Verification items for this drawing (mm, ordinates from the low corner). Coordinates: 2 decimals unless noted, no trailing zeros. One line per item, written item: value. Start each with the question number.
1) Scan lines: line 1 along Z through (x, y) = (170, 0.65); line 2 along X through (y, z) = (0.6, 115); line 3 along X through (y, z) = (1.5, 5). Record each from-to range of solid material in increasing order. Write a range as [from, to].
2) Gauge pin test, flat ends, axial feed: P1, Ø5, axis at x = 100.5, z = 70.5, coming from the -Y side; P2, Ø2.5, axis at x = 170, z = 115, coming from the +Y side. Record the tip position at first contact, or that the pin passes through.
3) Draft check along Y on the marked faces 1 and 2. Enter one of: +Y half, -Y half, draft (parallel to the pull), parting line (faces both ways), or undercut.
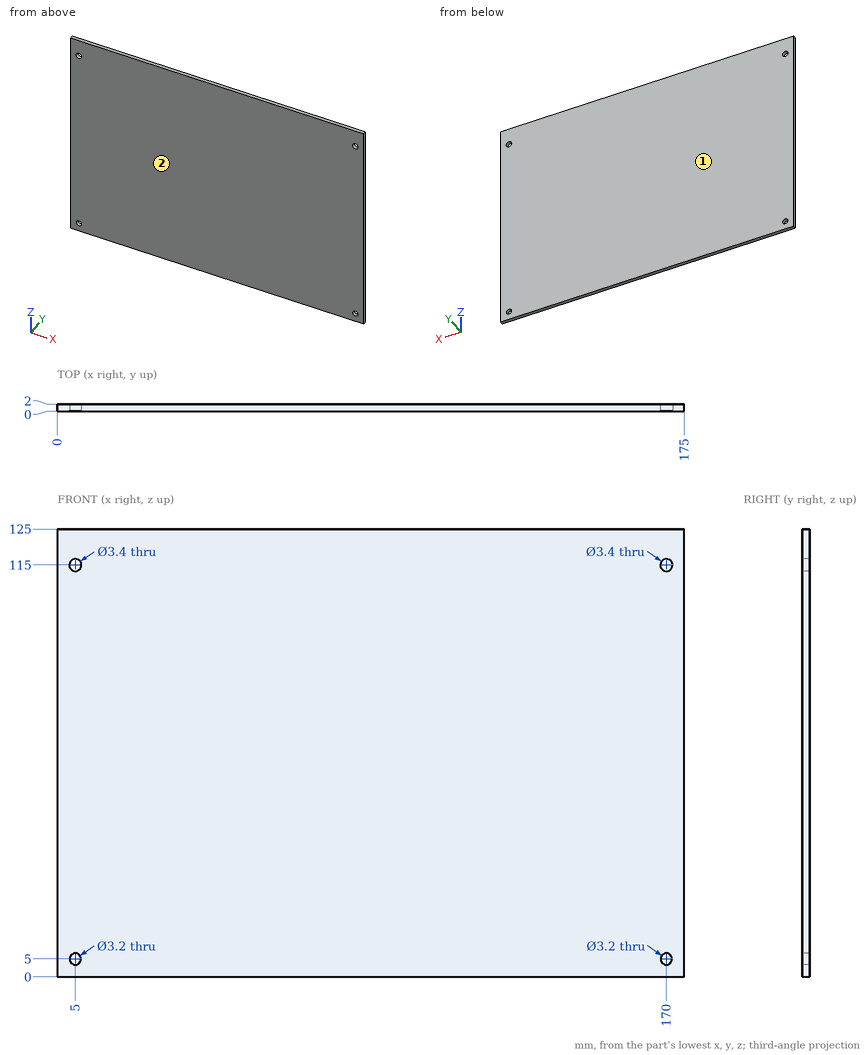
Answers:
1. line 1: z = [0, 3.4], [6.6, 113.3], [116.7, 125]
1. line 2: x = [0, 3.3], [6.7, 168.3], [171.7, 175]
1. line 3: x = [0, 3.4], [6.6, 168.4], [171.6, 175]
2. P1: stops at y = 0
2. P2: passes through
3. face 1: +Y half
3. face 2: -Y half
